from build123d import *

# Parameters (mm, degrees)
EXTRUDE_1_DEPTH            = 48
CUT_EXTRUDE_2_REACH        = 96.508
CUT_EXTRUDE_2_START_RADIUS = 70
CUT_EXTRUDE_2_END_RADIUS   = 70
SKETCH_3_W                 = 58.404028666
SKETCH_3_H                 = 6
EXTRUDE_2_DEPTH            = 13
CUT_EXTRUDE_3_DEPTH        = 140.034418617
CUT_EXTRUDE_3_DEPTH_BACK   = 140.034418617
SKETCH_4_W                 = 25
SKETCH_4_H                 = 38
SKETCH_4_W_2               = 40
SKETCH_4_H_2               = 25
CHAMFER_1_SIZE             = 5
CHAMFER_1_SIZE2            = 3.813196151
SKETCH_6_R                 = 6.5
CUT_EXTRUDE_4_DEPTH        = 2
SKETCH_7_R                 = 1.5
CUT_EXTRUDE_5_DEPTH        = 60
SKETCH_8_W                 = 9
SKETCH_8_H                 = 9
CUT_EXTRUDE_6_DEPTH        = 11
CUT_EXTRUDE_8_REACH        = 137.533
SKETCH_10_R                = 1
CUT_EXTRUDE_9_REACH        = 105.034
CUT_EXTRUDE_9_END_RADIUS   = 70
SKETCH_11_R                = 0.75
SKETCH_12_W                = 20
SKETCH_12_H                = 3
CUT_EXTRUDE_10_DEPTH       = 11
SKETCH_13_W                = 3.868283576
SKETCH_13_H                = 1.5
CUT_EXTRUDE_11_DEPTH       = 4
CUT_EXTRUDE_12_REACH       = 137.476
SKETCH_15_W                = 94.926723873
SKETCH_15_H                = 55.523178114
CUT_EXTRUDE_13_DEPTH       = 10


with BuildPart() as part:
    # 草图1 → 凸台-拉伸1 (new body)
    with BuildSketch(Plane(origin=(0, 0, 0), x_dir=(1, 0, 0), z_dir=(0, 1, 0))):
        with BuildLine():
            ThreePointArc((-9.396926208, -7.075874358), (-5.735764364, -11.847193368), (0, -13.655672925))
            Line((0, -13.655672925), (0, -5))
            ThreePointArc((0, -5), (-5, 0), (0, 5))
            Line((0, 5), (0, 70))
            ThreePointArc((0, 70), (-17.673593853, 67.732149533), (-34.202014333, 61.075545152))
            Line((-34.202014333, 61.075545152), (-9.396926208, -7.075874358))
        make_face()
        with BuildLine():
            Line((0, -5), (0, -13.655672925))
            ThreePointArc((0, -13.655672925), (5.735764364, -11.847193368), (9.396926208, -7.075874358))
            Line((9.396926208, -7.075874358), (34.202014333, 61.075545152))
            ThreePointArc((34.202014333, 61.075545152), (17.673593853, 67.732149533), (0, 70))
            Line((0, 70), (0, 5))
            ThreePointArc((0, 5), (3.535533906, 3.535533906), (5, 0))
            ThreePointArc((5, 0), (3.535533906, -3.535533906), (0, -5))
        make_face()
    extrude(amount=EXTRUDE_1_DEPTH)

    # 切除-拉伸2: from a cylinder face, 96.508 long prism both ways, kept between that surface and its translate by the depth
    cut_extrude_2_start = Plane(origin=(0, 5, 0), z_dir=(0, -1, 0)) * Cylinder(CUT_EXTRUDE_2_START_RADIUS, 334.016, mode=Mode.PRIVATE)
    cut_extrude_2_end = Plane(origin=(0, 5, 3), z_dir=(0, -1, 0)) * Cylinder(CUT_EXTRUDE_2_END_RADIUS, 334.016, mode=Mode.PRIVATE)
    # 草图3 → 切除-拉伸2 (cut, from a surface)
    with BuildSketch(Plane.XY, mode=Mode.PRIVATE) as cut_extrude_2_sk1:
        with Locations((3, 5)):
            Rectangle(SKETCH_3_W, SKETCH_3_H)
    cut_extrude_2_tool1 = extrude(cut_extrude_2_sk1.sketch, amount=CUT_EXTRUDE_2_REACH, both=True, mode=Mode.PRIVATE)
    add(((cut_extrude_2_tool1 & cut_extrude_2_start) - cut_extrude_2_end).solids().sort_by_distance((3, 5, -62.032204))[0], mode=Mode.SUBTRACT)

    # 草图2 → 凸台-拉伸2 (add)
    with BuildSketch(Plane(origin=(0, 48, 0), x_dir=(1, 0, 0), z_dir=(0, 1, 0))):
        Polygon((24.252642572, 33.739870901), (55.034455471, 118.312206771), (20.125623779, 80.877067961), (5.458790156, 40.580273767), align=None)
    extrude(amount=-EXTRUDE_2_DEPTH)

    # 草图4 → 切除-拉伸3 (cut, two sides: drawn at the far end of the back side and taken through both)
    with BuildSketch(Plane(origin=(0, 0, 0), x_dir=(0, 0, -1), z_dir=(1, 0, 0)).offset(-CUT_EXTRUDE_3_DEPTH_BACK)):
        with Locations((-1.155672925, 29)):
            Rectangle(SKETCH_4_W, SKETCH_4_H)
        with Locations((50.466884927, 22.5)):
            Rectangle(SKETCH_4_W_2, SKETCH_4_H_2)
    extrude(amount=CUT_EXTRUDE_3_DEPTH + CUT_EXTRUDE_3_DEPTH_BACK, mode=Mode.SUBTRACT)

    # 倒角1
    chamfer_1_edges = [part.edges().sort_by_distance(p)[0] for p in [
        (55.034455471, 41.5, -118.312206771),
    ]]
    chamfer_1_side = [part.faces().sort_by_distance(p)[0] for p in [
        (37.580039625, 41.5, -99.594637366),
    ]]
    chamfer(chamfer_1_edges, length=CHAMFER_1_SIZE, length2=CHAMFER_1_SIZE2, reference=chamfer_1_side[0])

    # 草图6 → 切除-拉伸4 (cut)
    with BuildSketch(Plane.XZ):
        with Locations(Location((0, 0, 0), (0, 0, 270))):
            Circle(SKETCH_6_R)
    extrude(amount=-CUT_EXTRUDE_4_DEPTH, mode=Mode.SUBTRACT)

    # 草图7 → 切除-拉伸5 (cut)
    with BuildSketch(Plane.XY):
        with Locations((-30.202014333, 5)):
            Circle(SKETCH_7_R)
    extrude(amount=-CUT_EXTRUDE_5_DEPTH, mode=Mode.SUBTRACT)

    # 草图8 → 切除-拉伸6 (cut)
    with BuildSketch(Plane(origin=(0, 10, 0), x_dir=(1, 0, 0), z_dir=(0, 1, 0))):
        with Locations((-30.258231885, 50.240091929)):
            Rectangle(SKETCH_8_W, SKETCH_8_H)
    extrude(amount=-CUT_EXTRUDE_6_DEPTH, mode=Mode.SUBTRACT)

    # 切除-拉伸8: up to this plane
    cut_extrude_8_end = Plane(origin=(32.202014333, 48, -62.153280468), z_dir=(-1, 0, 0))
    # 草图10 → 切除-拉伸8 (cut, up to the surface)
    with BuildSketch(Plane(origin=(10.571836839, 0, 3.847833931), x_dir=(0.34202014332566283, 0, -0.9396926207859106), z_dir=(0.9396926207859106, 0, 0.34202014332566283)), mode=Mode.PRIVATE) as cut_extrude_8_sk1:
        with Locations((67.590016934, 5)):
            Circle(SKETCH_10_R)
    cut_extrude_8_tool1 = split(extrude(cut_extrude_8_sk1.sketch, amount=-CUT_EXTRUDE_8_REACH, mode=Mode.PRIVATE), bisect_by=cut_extrude_8_end, keep=Keep.BOTH, mode=Mode.PRIVATE)
    add(cut_extrude_8_tool1.solids().sort_by_distance((33.688984, 5, -59.666006))[0], mode=Mode.SUBTRACT)

    # 切除-拉伸9: up to this cylinder (the profile starts inside it)
    cut_extrude_9_end = Plane(origin=(0, 5, 0), z_dir=(0, -1, 0)) * Cylinder(CUT_EXTRUDE_9_END_RADIUS, 351.068, mode=Mode.PRIVATE)
    # 草图11 → 切除-拉伸9 (cut, up to the surface)
    with BuildSketch(Plane.XY.offset(-60), mode=Mode.PRIVATE) as cut_extrude_9_sk1:
        with Locations((-30.202014333, 5)):
            Circle(SKETCH_11_R)
    cut_extrude_9_tool1 = extrude(cut_extrude_9_sk1.sketch, amount=-CUT_EXTRUDE_9_REACH, mode=Mode.PRIVATE) & cut_extrude_9_end
    add(cut_extrude_9_tool1.solids().sort_by_distance((-30.202014, 5, -60))[0], mode=Mode.SUBTRACT)

    # 草图12 → 切除-拉伸10 (cut)
    with BuildSketch(Plane(origin=(0, 10, 0), x_dir=(1, 0, 0), z_dir=(0, 1, 0))):
        with Locations((8.346963974, 51.411545488)):
            Rectangle(SKETCH_12_W, SKETCH_12_H)
    extrude(amount=-CUT_EXTRUDE_10_DEPTH, mode=Mode.SUBTRACT)

    # 草图13 → 切除-拉伸11 (cut)
    with BuildSketch(Plane(origin=(0, 10, 0), x_dir=(1, 0, 0), z_dir=(0, 1, 0))):
        with Locations((29.542762739, 51.411545488)):
            Rectangle(SKETCH_13_W, SKETCH_13_H)
    extrude(amount=-CUT_EXTRUDE_11_DEPTH, mode=Mode.SUBTRACT)

    # 草图14 → 切除-拉伸12 (cut, up to next)
    with BuildSketch(Plane(origin=(0, 48, 0), x_dir=(1, 0, 0), z_dir=(0, 1, 0)), mode=Mode.PRIVATE) as cut_extrude_12_sk1:
        Polygon((49.766128767, 108.223290792), (49.034775066, 108.905289152), (40.168796385, 99.397691031), (40.900150086, 98.715692671), align=None)
    cut_extrude_12_tool1 = extrude(cut_extrude_12_sk1.sketch, amount=-CUT_EXTRUDE_12_REACH, mode=Mode.PRIVATE) & part.part
    add(cut_extrude_12_tool1.solids().sort_by_distance((44.967463, 48, -103.810491))[0], mode=Mode.SUBTRACT)

    # 草图15 → 切除-拉伸13 (cut)
    with BuildSketch(Plane(origin=(0, 10, 0), x_dir=(1, 0, 0), z_dir=(0, 1, 0))):
        with Locations((-0.892742436, 58.228473984)):
            Rectangle(SKETCH_15_W, SKETCH_15_H)
    extrude(amount=-CUT_EXTRUDE_13_DEPTH, mode=Mode.SUBTRACT)


solid = part.part
Here's how the part is built. I have some questions about the finished solid (model axes, mm). A direction names the side the tool comes from. Round coordinates to 2 decimals unless told otherwise and drop trailing zeros. Write each loop counter-clockwise with the first axis right and the second up, starting at its lowest first coordinate (ties: lowest second). Pieces come first, ordered by that corner, then holes.
1. If we mould it in two halves opening along Z, with no side actions, what happens to faces 5 (the flat face through (45.27, 41.59, -103.4)), 6 (the flat face through (0, 18, -30.467)), 7 (the flat face through (9, 48, -52)), 8 (the flat face through (0, 29, -11.344))? For each: released by +Z, released by -Z, zero draft, split by the parting line, or undercut.
2. Will these pins go through, and if not, where does the flat tip stop? pin 1 Ø3 at (x, z) = (11.5, -37) entering from -Y; pin 2 Ø6.5 at (x, z) = (-2, -3) entering from -Y; pin 3 Ø4 at (y, z) = (10.5, -12.5) entering from +X; pin 4 Ø10.5 at (x, y) = (0.5, 12.5) entering from -Z.
3. I need wall thicknesses on L1, parallel to Y at x = 16, z = -57.5; L2, parallel to X at y = 0.5, z = 0; L3, parallel to Z at x = 9, y = 34. Which ranges of each line are inside material? Lowest first, please.
4. For faces 1 (the cylindrical face through (-3.955, 0.986, 5.158)), 2 (the flat face through (3.4, 10, -4.2)), 3 (the flat face through (44.664, 41.591, -104.218)), 4 (the flat face through (9, 35, -63)), which set-ups out of +Z, -Z, +X, -X, +Y, -Y let a thin tool reach every point of the face, with its end or its side?
5. Suppose I cut it at C-C (x = 29). List the corners of the cut face in (y, z) for me, and give its area (3 significant figures).
6. Suppose I cut it at D-D (x = -17.5). List the corners of the cut face in (y, z) for me, and give its area (3 significant figures).
7. Suppose I cut it at A-A (z = -106). List the corners of the cut face in (x, y) for me.
8. Suppose I cut it at B-B (y = 14). List the corners of the cut face in (x, z) for me, and give its area (3 significant figures).
Answer sheet:
1. face 5: undercut
1. face 6: released by -Z
1. face 7: zero draft
1. face 8: released by +Z
2. pin 1: stops at y = 35
2. pin 2: stops at y = 0
2. pin 3: stops at x = 17.25
2. pin 4: stops at z = -30.47
3. L1: y = 35 to 48
3. L2: x = -11.97 to -6.5, 6.5 to 11.97
3. L3: z = -30.47 to -11.34
4. face 1: -Y
4. face 2: +Z, +X, -X, +Y
4. face 3: +Y, -Y
4. face 4: -Z, +X, -X, -Y
5. outline: (35, -90.39) - (48, -90.39) - (48, -46.78) - (35, -46.78) - close
5. area: 567 mm2
6. outline: (0, -30.47) - (35, -30.47) - (35, -67.78) - (48, -67.78) - (48, -15.19) - (0, -15.19) - close
6. area: 1,220 mm2
7. outline: (43.55, 35) - (46.33, 35) - (46.33, 48) - (43.55, 48) - close; (47.69, 35) - (50.55, 35) - (50.55, 48) - (47.69, 48) - close
8. outline: (-23.06, -30.47) - (23.06, -30.47) - (16.1, -11.34) - (-16.1, -11.34) - close
8. area: 749 mm2
